```python
from build123d import *

# Parameters (mm, degrees)
F0_W     = 50.8
F0_H     = 50.8
F1_DEPTH = 12.7
F2_SIZE  = 12.7
F3_T     = -1.524


with BuildPart() as f1:
    # F0 (on Front) → F1 (new body, symmetric)
    with BuildSketch(Plane.XZ):
        with Locations((0, 25.4)):
            Rectangle(F0_W, F0_H)
    extrude(amount=F1_DEPTH, both=True)

    # F2
    f2_edges = [f1.edges().sort_by_distance(p)[0] for p in [
        (-25.4, 0, 0),
        (25.4, 0, 0),
    ]]
    chamfer(f2_edges, length=F2_SIZE)

    # F3
    f3_openings = [f1.faces().sort_by_distance(p)[0] for p in [
        (0, 0, 50.8),
        (0, 0, 0),
    ]]
    offset(amount=F3_T, openings=f3_openings)


solid = f1.part
```
Geometry: final body of the model. Coordinates: model frame, mm. A direction names the side the tool comes from. Round coordinates to 2 decimals unless told otherwise and drop trailing zeros. Write each loop counter-clockwise with the first axis right and the second up, starting at its lowest first coordinate (ties: lowest second). Pieces come first, ordered by that corner, then holes.
Item 1: Section query A-A (x = -5.5). Return loops of the section in (y, z).
Item 2: Section query B-B (z = 20.5). Return loops of the section in (x, y).
Item 3: Section query D-D (x = -16). Return loops of the section in (y, z).
Item 4: Pin query (flat end, axial travel): P1, Ø1, axis at y = 5, z = 5.5, coming from the -X side. Return the tip coordinate at first contact, or that it passes through.
Item 5: Mould query, pull axis Y, two halves, no side actions, for faces 3 (the face through (0, -12.7, 26)), 4 (the face through (0, -11.176, 26)), 5 (the face through (0, 12.7, 26)), 6 (the face through (0, 12, 50.8)). Classes: +Y half, -Y half, draft (parallel to the pull), parting line (faces both ways), or undercut.
Item 6: Material intervals for L1, parallel to Y at x = 0, z = 47.5; L2, parallel to X at y = -10, z = 34; L3, parallel to X at y = 1.5, z = 2, sorted ascending.
Item 7: Set-up query: faces 1 (the face through (23.876, 0, 32)), 2 (the face through (-25.4, 0, 31)). Return all of +Z, -Z, +X, -X, +Y, -Y with unobstructed straight access to the full face (end or side cutting, diameter ignored); none if empty.
Item 8: Section query C-C (y = 0.5). Return loops of the section in (x, z).
Completed:
1. outline: (-12.7, 0) - (-11.18, 0) - (-11.18, 50.8) - (-12.7, 50.8) - close; (11.18, 0) - (12.7, 0) - (12.7, 50.8) - (11.18, 50.8) - close
2. outline: (-25.4, -12.7) - (25.4, -12.7) - (25.4, 12.7) - (-25.4, 12.7) - close; hole (-23.88, -11.18) - (23.88, -11.18) - (23.88, 11.18) - (-23.88, 11.18) - close
3. outline: (-12.7, 3.3) - (12.7, 3.3) - (12.7, 50.8) - (11.18, 50.8) - (11.18, 5.46) - (-11.18, 5.46) - (-11.18, 50.8) - (-12.7, 50.8) - close
4. P1: stops at x = -18.7
5. face 3: -Y half
5. face 4: undercut
5. face 5: +Y half
5. face 6: draft
6. L1: y = -12.7 to -11.18, 11.18 to 12.7
6. L2: x = -25.4 to -23.88, 23.88 to 25.4
6. L3: x = -14.7 to -12.54, 12.54 to 14.7
7. face 1: +Z
7. face 2: +Z, -Z, -X, +Y, -Y
8. outline: (-25.4, 12.7) - (-12.7, 0) - (-10.54, 0) - (-23.88, 13.33) - (-23.88, 50.8) - (-25.4, 50.8) - close; (10.54, 0) - (12.7, 0) - (25.4, 12.7) - (25.4, 50.8) - (23.88, 50.8) - (23.88, 13.33) - close
